Job drawing, mm, ordinate dimensions from the low corner. One solid piece. A direction names the side the tool comes from. Round coordinates to 2 decimals unless told otherwise and drop trailing zeros. Write each loop counter-clockwise with the first axis right and the second up, starting at its lowest first coordinate (ties: lowest second). Pieces come first, ordered by that corner, then holes. Notation, with made-up numbers: (-16.5, 27) -> (20.5, 27) arc R31 ccw to (20.5, 65) -> close; hole circle Ø10 at (89.25, 6). An arc over 180 degrees is marked (long way). Use CSV: the item, a comma, the result in double quotes. Start each with the question number.
(1) Two-plate mould, pull along Z, no slides. Class the marked faces 1, 2 and 3: released by +Z, released by -Z, zero draft, split by the parting line, or undercut.
(2) Which spindle directions (+Z, -Z, +X, -X, +Y, -Y) get a long thin tool onto all of the face, cutting with end or side? Do the marked faces 4, 5, 6 and 7. Say none if no direction does.
(3) Saw through at B-B (y = 23). Give the cut face in (x, z).
(4) Drop flat-ended pins along their axis: pin 1 (2 mm diameter, centred on x = 2.5, z = 16.5, fed in from -Y); pin 2 (4 mm diameter, centred on y = 7, z = 15.5, fed in from -X); pin 3 (2.5 mm diameter, centred on x = 5, z = 14.5, fed in from +Y); pin 4 (6 mm diameter, centred on x = 27.9, z = 16, fed in from -Y). Give the stop position or say it passes through.
(5) Saw through at D-D (z = 10). Give the cut face in (x, y).
(6) Saw through at C-C (x = 34.5). Give the cut face in (y, z) (1 decimal).
(7) Probe line 1 (Z direction, x = 27.9, y = 3); line 2 (X direction, y = 4.25, z = 16); line 3 (Z direction, x = 17, y = 15). List the from-to ranges inside material, lowest first. Write a range as [from, to].
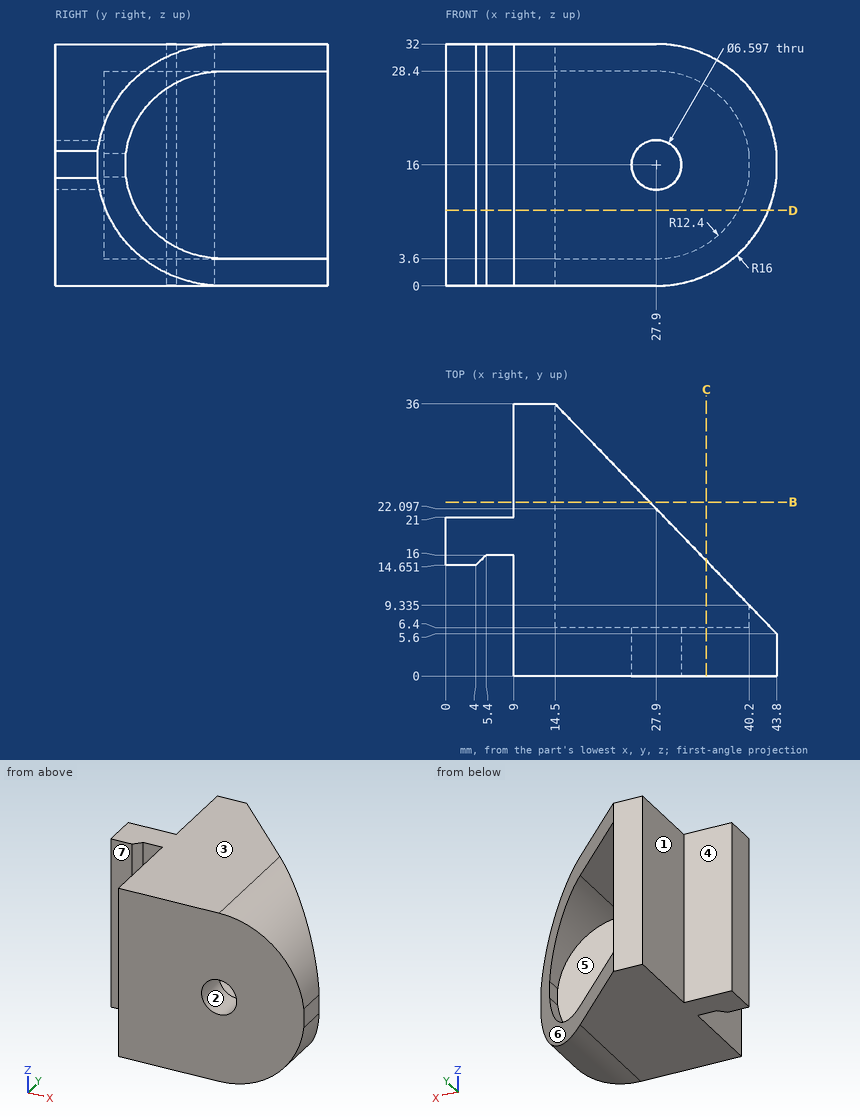
Answers:
1,face 1,"zero draft"
1,face 2,"undercut"
1,face 3,"released by +Z"
2,face 4,"+Z, -Z, -X, +Y"
2,face 5,"+Y"
2,face 6,"+Z, -Z, +X, +Y"
2,face 7,"+Z, -Z, -X, -Y"
3,outline,"(9, 0) -> (27.03, 0) -> (27.03, 3.6) -> (14.5, 3.6) -> (14.5, 28.4) -> (27.03, 28.4) -> (27.03, 32) -> (9, 32) -> close"
4,pin 1,"stops at y = 14.65"
4,pin 2,"stops at x = 9"
4,pin 3,"stops at y = 21"
4,pin 4,"passes through"
5,outline,"(0, 14.65) -> (4, 14.65) -> (5.4, 16) -> (9, 16) -> (9, 0) -> (42.73, 0) -> (42.73, 6.71) -> (38.75, 10.84) -> (38.75, 6.4) -> (14.5, 6.4) -> (14.5, 36) -> (9, 36) -> (9, 21) -> (0, 21) -> close"
6,outline,"(0, 1.4) -> (15.2, 1.4) -> (15.2, 5.5) -> (6.4, 5.5) -> (6.4, 26.5) -> (15.2, 26.5) -> (15.2, 30.6) -> (0, 30.6) -> close"
7,line 1,"z = [0, 12.7], [19.3, 32]"
7,line 2,"x = [9, 24.6], [31.2, 43.8]"
7,line 3,"z = [0, 3.6], [28.4, 32]"
